from build123d import *

# Parameters (mm, degrees)
SKETCH_1_W                     = 166
SKETCH_1_H                     = 138
EXTRUDE_1_DEPTH                = 2
EXTRUDE_2_DEPTH                = 6
EXTRUDE_2_DEPTH_BACK           = 14
SKETCH_2_W                     = 158
SKETCH_2_H                     = 130
SKETCH_2_W_2                   = 154
SKETCH_2_H_2                   = 126
SKETCH_3_R                     = 1.5
EXTRUDE_2_2_DEPTH              = 5
SKETCH_5_R                     = 1.5
EXTRUDE_3_DEPTH                = 5
SKETCH_4_R                     = 1.5
EXTRUDE_4_DEPTH                = 5
SKETCH_6_W                     = 75
SKETCH_6_H                     = 2
SKETCH_6_W_2                   = 2
SKETCH_6_H_2                   = 75
EXTRUDE_5_DEPTH                = 8
SKETCH_9_W                     = 90
SKETCH_9_H                     = 2
EXTRUDE_6_DEPTH                = 1
FILLET_1_R                     = 1
SKETCH_11_W                    = 90
SKETCH_11_H                    = 2
EXTRUDE_7_DEPTH                = 1
FILLET_2_R                     = 1
PATTERN_LINEAR_1_COUNT         = 2
PATTERN_LINEAR_1_PITCH         = 8
FILLET_1_OF_PATTERN_LINEAR_1_R = 1
PATTERN_LINEAR_2_COUNT         = 2
PATTERN_LINEAR_2_PITCH         = 8
FILLET_2_OF_PATTERN_LINEAR_2_R = 1
SKETCH_12_W                    = 2
SKETCH_12_H                    = 12
SKETCH_12_W_2                  = 12
SKETCH_12_H_2                  = 2
SKETCH_12_H_3                  = 1.3
EXTRUDE_8_DEPTH                = 8
CUT_EXTRUDE_2_DEPTH            = 109.839331126
CUT_EXTRUDE_2_DEPTH_BACK       = 109.839331126
SKETCH_5_4_R                   = 1.5
CUT_EXTRUDE_3_DEPTH            = 109.839331126
CUT_EXTRUDE_3_DEPTH_BACK       = 109.839331126
SKETCH_4_3_R                   = 1.5
CUT_EXTRUDE_4_DEPTH            = 109.839331126
CUT_EXTRUDE_4_DEPTH_BACK       = 109.839331126
SKETCH_3_2_R                   = 1.5
SKETCH_13_R                    = 3
SKETCH_13_R_2                  = 4
CUT_EXTRUDE_5_DEPTH            = 109.839331126


with BuildPart() as part:
    # 스케치1 → 보스-돌출1 (new body)
    with BuildSketch(Plane.XY):
        Rectangle(SKETCH_1_W, SKETCH_1_H)
    extrude(amount=EXTRUDE_1_DEPTH)

    # 스케치2 → Extrude 2 (add, two sides: drawn at the far end of the back side and taken through both)
    with BuildSketch(Plane.XY.offset(2).offset(-EXTRUDE_2_DEPTH_BACK)):
        Rectangle(SKETCH_2_W, SKETCH_2_H)
        Rectangle(SKETCH_2_W_2, SKETCH_2_H_2, mode=Mode.SUBTRACT)
    extrude(amount=EXTRUDE_2_DEPTH + EXTRUDE_2_DEPTH_BACK)

    # 스케치3 → Extrude 2 2 (add)
    with BuildSketch(Plane.XY.offset(2)):
        with Locations(Location((-65, -42, 0), (0, 0, 180))):
            Circle(SKETCH_3_R)
        with Locations(Location((-50, -42, 0), (0, 0, 180))):
            Circle(SKETCH_3_R)
        with Locations(Location((-65, 42, 0), (0, 0, 180))):
            Circle(SKETCH_3_R)
        with Locations(Location((-50, 42, 0), (0, 0, 180))):
            Circle(SKETCH_3_R)
    extrude(amount=EXTRUDE_2_2_DEPTH)

    # 스케치5 → 보스-돌출3 (add)
    with BuildSketch(Plane.XY.offset(2)):
        with Locations(Location((42, 56, 0), (0, 0, 180))):
            Circle(SKETCH_5_R)
        with Locations(Location((42, 41, 0), (0, 0, 180))):
            Circle(SKETCH_5_R)
    extrude(amount=EXTRUDE_3_DEPTH)

    # 스케치4 → 보스-돌출4 (add)
    with BuildSketch(Plane.XY.offset(2)):
        with Locations(Location((-42, 56, 0), (0, 0, 180))):
            Circle(SKETCH_4_R)
        with Locations(Location((-42, 41, 0), (0, 0, 180))):
            Circle(SKETCH_4_R)
    extrude(amount=EXTRUDE_4_DEPTH)

    # 스케치6 → 보스-돌출5 (add)
    with BuildSketch(Plane.XY.offset(2)):
        with Locations((0, -54)):
            Rectangle(SKETCH_6_W, SKETCH_6_H)
        with Locations((0, -44)):
            Rectangle(SKETCH_6_W, SKETCH_6_H)
        with Locations((46, 0)):
            Rectangle(SKETCH_6_W_2, SKETCH_6_H_2)
        with Locations((56, 0)):
            Rectangle(SKETCH_6_W_2, SKETCH_6_H_2)
    extrude(amount=EXTRUDE_5_DEPTH)

    # 스케치9 → 보스-돌출6 (add)
    with BuildSketch(Plane.XZ.offset(65)):
        with Locations((0, 5)):
            Rectangle(SKETCH_9_W, SKETCH_9_H)
    extrude_6 = extrude(amount=EXTRUDE_6_DEPTH)

    # 필렛1
    fillet_1_edges = [part.edges().sort_by_distance(p)[0] for p in [
        (0, -66, 4),
        (0, -66, 6),
    ]]
    fillet(fillet_1_edges, radius=FILLET_1_R - 0.0001)  # a hair under: the kernel refuses the full size

    # 스케치11 → 보스-돌출7 (add)
    with BuildSketch(Plane(origin=(0, 65, 0), x_dir=(1, 0, 0), z_dir=(0, 1, 0))):
        with Locations((0, -5)):
            Rectangle(SKETCH_11_W, SKETCH_11_H)
    extrude_7 = extrude(amount=EXTRUDE_7_DEPTH)

    # 필렛2
    fillet_2_edges = [part.edges().sort_by_distance(p)[0] for p in [
        (0, 66, 4),
        (0, 66, 6),
    ]]
    fillet(fillet_2_edges, radius=FILLET_2_R - 0.0001)  # a hair under: the kernel refuses the full size

    # 선형 패턴1: 보스-돌출6 ×2
    with Locations(*[(0, 0, -i * PATTERN_LINEAR_1_PITCH) for i in range(1, PATTERN_LINEAR_1_COUNT)]):
        add(extrude_6)

    # 필렛1 of 선형 패턴1
    fillet_1_of_pattern_linear_1_edges = [part.edges().sort_by_distance(p)[0] for p in [
        (0, -66, -4),
        (0, -66, -2),
    ]]
    fillet(fillet_1_of_pattern_linear_1_edges, radius=FILLET_1_OF_PATTERN_LINEAR_1_R - 0.0001)  # a hair under: the kernel refuses the full size

    # 선형 패턴2: 보스-돌출7 ×2
    with Locations(*[(0, 0, -i * PATTERN_LINEAR_2_PITCH) for i in range(1, PATTERN_LINEAR_2_COUNT)]):
        add(extrude_7)

    # 필렛2 of 선형 패턴2
    fillet_2_of_pattern_linear_2_edges = [part.edges().sort_by_distance(p)[0] for p in [
        (0, 66, -4),
        (0, 66, -2),
    ]]
    fillet(fillet_2_of_pattern_linear_2_edges, radius=FILLET_2_OF_PATTERN_LINEAR_2_R - 0.0001)  # a hair under: the kernel refuses the full size

    # 스케치12 → 보스-돌출8 (add)
    with BuildSketch(Plane.XY.offset(2)):
        with Locations((-38.5, -49)):
            Rectangle(SKETCH_12_W, SKETCH_12_H)
        with Locations((38.5, -49)):
            Rectangle(SKETCH_12_W, SKETCH_12_H)
        with Locations((51, -38.5)):
            Rectangle(SKETCH_12_W_2, SKETCH_12_H_2)
        with Locations((51, 38.15)):
            Rectangle(SKETCH_12_W_2, SKETCH_12_H_3)
    extrude(amount=EXTRUDE_8_DEPTH)

    # 스케치5<4> → 컷-돌출2 (cut, two sides: drawn at the far end of the back side and taken through both)
    with BuildSketch(Plane.XY.offset(2).offset(-CUT_EXTRUDE_2_DEPTH_BACK)):
        with Locations(Location((42, 56, 0), (0, 0, 180))):
            Circle(SKETCH_5_4_R)
        with Locations(Location((42, 41, 0), (0, 0, 180))):
            Circle(SKETCH_5_4_R)
    extrude(amount=CUT_EXTRUDE_2_DEPTH + CUT_EXTRUDE_2_DEPTH_BACK, mode=Mode.SUBTRACT)

    # 스케치4<3> → 컷-돌출3 (cut, two sides: drawn at the far end of the back side and taken through both)
    with BuildSketch(Plane.XY.offset(2).offset(-CUT_EXTRUDE_3_DEPTH_BACK)):
        with Locations(Location((-42, 56, 0), (0, 0, 180))):
            Circle(SKETCH_4_3_R)
        with Locations(Location((-42, 41, 0), (0, 0, 180))):
            Circle(SKETCH_4_3_R)
    extrude(amount=CUT_EXTRUDE_3_DEPTH + CUT_EXTRUDE_3_DEPTH_BACK, mode=Mode.SUBTRACT)

    # 스케치3<2> → 컷-돌출4 (cut, two sides: drawn at the far end of the back side and taken through both)
    with BuildSketch(Plane.XY.offset(2).offset(-CUT_EXTRUDE_4_DEPTH_BACK)):
        with Locations(Location((-65, -42, 0), (0, 0, 180))):
            Circle(SKETCH_3_2_R)
        with Locations(Location((-50, -42, 0), (0, 0, 180))):
            Circle(SKETCH_3_2_R)
        with Locations(Location((-65, 42, 0), (0, 0, 180))):
            Circle(SKETCH_3_2_R)
        with Locations(Location((-50, 42, 0), (0, 0, 180))):
            Circle(SKETCH_3_2_R)
    extrude(amount=CUT_EXTRUDE_4_DEPTH + CUT_EXTRUDE_4_DEPTH_BACK, mode=Mode.SUBTRACT)

    # 스케치13 → 컷-돌출5 (cut, through all)
    with BuildSketch(Plane.XY.offset(2)):
        Circle(SKETCH_13_R)
        with Locations((-69, 55)):
            Circle(SKETCH_13_R_2)
        with Locations(Location((69, 55, 0), (0, 0, 180))):
            Circle(SKETCH_13_R_2)
        with Locations((69, -55)):
            Circle(SKETCH_13_R_2)
        with Locations((69, 0)):
            Circle(SKETCH_13_R_2)
    extrude(amount=-CUT_EXTRUDE_5_DEPTH, mode=Mode.SUBTRACT)


solid = part.part
The model under review builds one solid part; all positions refer to its coordinate system, in mm. A direction names the side the tool comes from. Round coordinates to 2 decimals unless told otherwise and drop trailing zeros. Loops run counter-clockwise (first coordinate to the right, second up) from the corner with the lowest first, then second, coordinate; pieces in that order, holes last. Notation, with made-up numbers: M 52.25,84 L 79.25,84 A34 ccw 79.25,117 Z; hole C -32.5,26 d1. An arc over 180 degrees is marked long. Answer as CSV lines item,"result".
1. We need section A-A (x = -69). Give the boundary of the cut face in (y, z).
Outcome:
outline,"M -69,0 L -65,0 L -65,-12 L -63,-12 L -63,0 L 51,0 L 51,2 L -63,2 L -63,8 L -65,8 L -65,2 L -69,2 Z; M 59,0 L 63,0 L 63,-12 L 65,-12 L 65,0 L 69,0 L 69,2 L 65,2 L 65,8 L 63,8 L 63,2 L 59,2 Z"
2. Draft analysis for pull direction X (two halves, no side actions). For faces 4 (the face through (-7, -66, 0)), 5 (the face through (-77, -1, -6)), 6 (the face through (-79, -1, 5)), state which applies: pulls with the +X half, pulls with the -X half, needs draft (parallel to the pull), parting line crosses it, or undercut.
Outcome:
face 4,"needs draft"
face 5,"undercut"
face 6,"pulls with the -X half"
3. Insertion check: pin 1 Ø8 at (x, y) = (-63.5, -6) entering from -Z; pin 2 Ø6.5 at (y, z) = (9, 6.5) entering from +X; pin 3 Ø6.5 at (x, z) = (51, 6) entering from -Y. Each pin has a flat end and moves straight along its axis. Give the tip position at first contact, or say it passes through.
Outcome:
pin 1,"stops at z = 0"
pin 2,"stops at x = 79"
pin 3,"stops at y = -65"
4. We need section D-D (y = 35.5). Give the boundary of the cut face in (x, z).
Outcome:
outline,"M -83,0 L -79,0 L -79,-12 L -77,-12 L -77,0 L 77,0 L 77,-12 L 79,-12 L 79,0 L 83,0 L 83,2 L 79,2 L 79,8 L 77,8 L 77,2 L 57,2 L 57,10 L 55,10 L 55,2 L 47,2 L 47,10 L 45,10 L 45,2 L -77,2 L -77,8 L -79,8 L -79,2 L -83,2 Z"
5. To check wall thickness, follow L1, parallel to Y at x = 69, z = 0.7; L2, parallel to Y at x = -50, z = 1.1; L3, parallel to Y at x = 12.5, z = 2.25. State the ranges of each line that lie inside material, in increasing order. Write a range as [from, to].
Outcome:
L1,"y = [-69, -59], [-51, -4], [4, 51], [59, 69]"
L2,"y = [-69, -43.5], [-40.5, 40.5], [43.5, 69]"
L3,"y = [-65, -63], [-55, -53], [-45, -43], [63, 65]"
6. We need section C-C (x = 69). Count the separate pieces of the cut face and the enclosed holes in it, plus the area to 3 significant figures.
Outcome:
separate pieces,"4"
enclosed holes,"0"
area,"300 mm2"
7. For faces 1 (the face through (-0.2, -44.5, 10)), 2 (the face through (-1, -63, -6)), 3 (the face through (51, 37.5, 6)), list the 3-axis set-ups (+Z, -Z, +X, -X, +Y, -Y) from which the entire face can be reached by the end or side of a thin tool; tool diameter is ignored.
Outcome:
face 1,"+Z, +X, -X, +Y, -Y"
face 2,"-Z"
face 3,"+Z"
8. We need section B-B (z = -10). Give the boundary of the cut face in (x, y), plus the area to 3 significant figures.
Outcome:
outline,"M -79,-65 L 79,-65 L 79,65 L -79,65 Z; hole M -77,-63 L 77,-63 L 77,63 L -77,63 Z"
area,"1,140 mm2"
